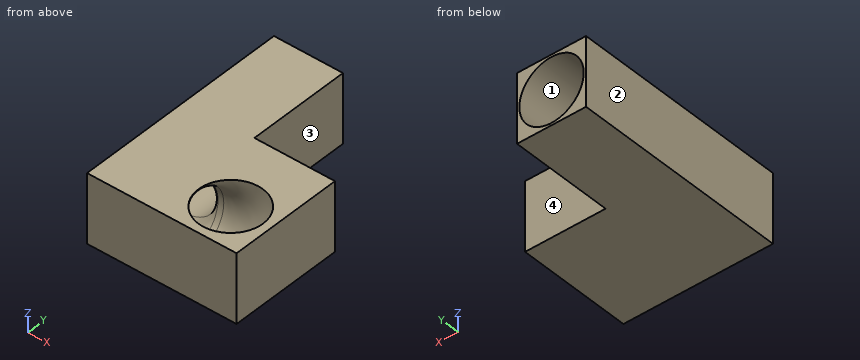
```python
from build123d import *

# Parameters (mm, degrees)
BOSS_EXTRUDE1_DEPTH = 76.2
SKETCH2_R           = 35.56


with BuildPart() as part:
    # Sketch1 → Boss-Extrude1 (new body)
    with BuildSketch(Plane.XY):
        Polygon((0, 241.3), (0, 0), (165.1, 0), (165.1, 127), (76.2, 127), (76.2, 241.3), align=None)
    extrude(amount=BOSS_EXTRUDE1_DEPTH)

    # Cut-Sweep1: sweep along a curve in space
    with BuildLine() as cut_sweep1_path:
        Line((38.1, 241.3, 38.1), (38.1, 82.55, 38.1))
        ThreePointArc((38.1, 82.55, 38.1), (49.259231637, 55.609231637, 38.1), (76.2, 44.45, 38.1))
        Line((76.2, 44.45, 38.1), (82.55, 44.45, 38.1))
        ThreePointArc((120.65, 44.45, 76.2), (109.490768363, 44.45, 49.259231637), (82.55, 44.45, 38.1))
    # Sketch2 → Cut-Sweep1 (sweep, cut)
    with BuildSketch(Plane(origin=(0, 241.3, 0), x_dir=(1, 0, 0), z_dir=(0, 1, 0))):
        with Locations((38.1, -38.1)):
            Circle(SKETCH2_R)
    sweep(path=cut_sweep1_path.line, mode=Mode.SUBTRACT)


solid = part.part
```
Here's how the part is built. I have some questions about the finished solid (model axes, mm). Face numbers are marked on the shaded views. Round coordinates to 2 decimals unless told otherwise and drop trailing zeros. Loops run counter-clockwise (first coordinate to the right, second up) from the corner with the lowest first, then second, coordinate; pieces in that order, holes last.
1. Thinking about a two-plate mould opening in X: for the marked faces 1, 2, 3 and 4, which applies, released by +X, released by -X, zero draft, split by the parting line, or undercut?
Answers:
face 1: undercut
face 2: released by -X
face 3: released by +X
face 4: zero draft
2. Will these pins go through, and if not, where does the flat tip stop? pin 1 (2 mm diameter, centred on x = 136, y = 63, fed in from +Z); pin 2 (4 mm diameter, centred on y = 158, z = 16, fed in from +X).
Answers:
pin 1: stops at z = 35.1
pin 2: stops at x = 76.2
3. Suppose I cut it at A-A, the plane y = 136.5. Please give me the cut outline in (x, z).
Answers:
outline: (0, 0) - (76.2, 0) - (76.2, 76.2) - (0, 76.2) - close; hole circle Ø71.12 at (38.1, 38.1)
4. If I drill on probe 1 along Z at (x, y) = (38, 121); probe 2 along X at (y, z) = (173, 39); probe 3 along Z at (x, y) = (52, 60.5), over which ranges is the centre line in solid material (lowest first)?
Answers:
probe 1: z = 0 to 2.54, 73.66 to 76.2
probe 2: x = 0 to 2.55, 73.65 to 76.2
probe 3: z = 0 to 2.95, 73.25 to 76.2
